The figure shows three views and two pictorial views of one solid part (mm, origin at its lowest corner). Answer the questions. A direction names the side the tool comes from. Coordinates: 2 decimals unless noted, no trailing zeros. Write each loop counter-clockwise with the first axis right and the second up, starting at its lowest first coordinate (ties: lowest second). Pieces come first, ordered by that corner, then holes. Notation, with made-up numbers: M -27.75,87.25 L -6.75,87.25 A23 ccw -6.75,103.25 Z; hole C -24,-38.75 d2. An arc over 180 degrees is marked long. Use CSV: the item, a comma, the result in double quotes.
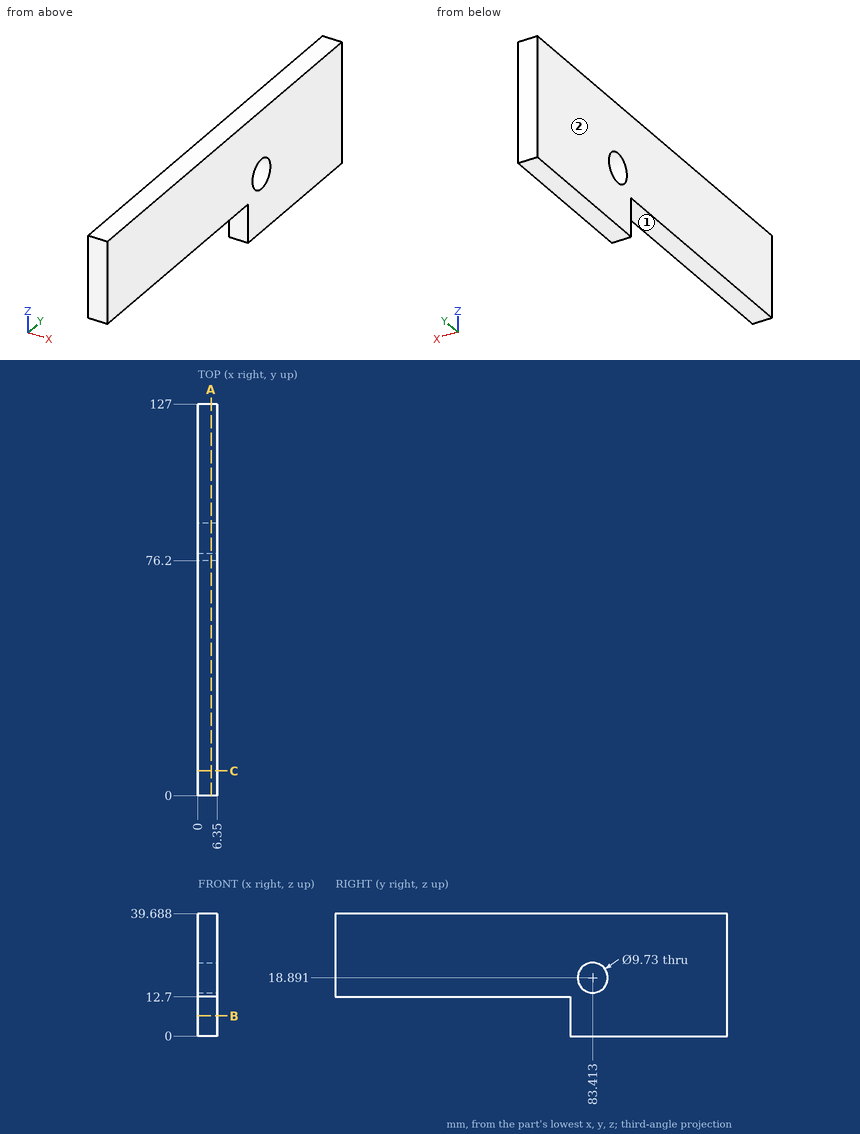
Item 1: Given pin 1 (6 mm diameter, centred on y = 83.41, z = 18.89, fed in from -X); pin 2 (1 mm diameter, centred on x = 5.5, z = 15.5, fed in from -Y); pin 3 (1 mm diameter, centred on x = 1.5, z = 5, fed in from -Y); pin 4 (1.9 mm diameter, centred on x = 2.5, y = 50, fed in from -Z), each flat-ended and moving along its own axis, determine where each tip first touches the part or whether it passes through.
Answer:
pin 1,"passes through"
pin 2,"stops at y = 0"
pin 3,"stops at y = 76.2"
pin 4,"stops at z = 12.7"
Item 2: The part is cut by section B-B (z = 6.5). Write down the section's boundary in (x, y).
Answer:
outline,"M 0,76.2 L 6.35,76.2 L 6.35,127 L 0,127 Z"
Item 3: Consider probe 1 along Z at (x, y) = (4, 83.5) (1 decimal); probe 2 along Y at (x, z) = (4, 11.5); probe 3 along Z at (x, y) = (3, 8). Determine where each line is inside the solid, lowest interval first.
Answer:
probe 1,"z = 0 to 14, 23.8 to 39.7"
probe 2,"y = 76.2 to 127"
probe 3,"z = 12.7 to 39.69"
Item 4: The part is cut by section C-C (y = 8). Write down the section's boundary in (x, z), then the cut area to 3 significant figures.
Answer:
outline,"M 0,12.7 L 6.35,12.7 L 6.35,39.69 L 0,39.69 Z"
area,"171 mm2"
Item 5: The part is cut by section A-A (x = 4.25). Write down the section's boundary in (y, z) (1 decimal).
Answer:
outline,"M 0,12.7 L 76.2,12.7 L 76.2,0 L 127,0 L 127,39.7 L 0,39.7 Z; hole C 83.4,18.9 d9.7"
Item 6: A tool of negligible diameter and unlimited length cuts with its end or side. For the marked faces 1 and 2, from which of +Z, -Z, +X, -X, +Y, -Y can it reach the whole face along a straight path? Write none if from no direction.
Answer:
face 1,"-Z, +X, -X, -Y"
face 2,"+Z, -Z, -X, +Y, -Y"
